from build123d import *

# Parameters (mm, degrees)
F0_R     = 2.1
F1_DEPTH = 19
F2_R     = 9.5
F3_DEPTH = 29.001
F4_R     = 5
F5_DEPTH = 38.001
F6_W     = 74.916892
F6_H     = 3.990418
F7_DEPTH = 29.001
F8_R     = 5
F9_DEPTH = 38.001


with BuildPart() as f1:
    # F0 (on Top) → F1 (new body)
    with BuildSketch(Plane.XY):
        Polygon((14, 14.5), (-14, 14.5), (-19, 9.5), (-19, -14.5), (19, -14.5), (19, 9.5), align=None)
        with Locations((-13, -9.8)):
            Circle(F0_R, mode=Mode.SUBTRACT)
        with Locations((13, -9.8)):
            Circle(F0_R, mode=Mode.SUBTRACT)
        with Locations((-13, 8.2)):
            Circle(F0_R, mode=Mode.SUBTRACT)
        with Locations((13, 8.2)):
            Circle(F0_R, mode=Mode.SUBTRACT)
    extrude(amount=F1_DEPTH)

    # F2 (on face) → F3 (cut, through all)
    with BuildSketch(Plane.XZ.offset(14.5)):
        with Locations((0, 16.5)):
            Circle(F2_R)
    extrude(amount=-F3_DEPTH, mode=Mode.SUBTRACT)

    # F4 (on face) → F5 (cut, through all)
    with BuildSketch(Plane.YZ.offset(19)):
        with Locations((-0.8, 0.2)):
            Circle(F4_R)
    extrude(amount=-F5_DEPTH, mode=Mode.SUBTRACT)

    # F6 (on face) → F7 (cut, through all)
    with BuildSketch(Plane.XZ.offset(14.5)):
        with Locations((0.39847, 18.995209)):
            Rectangle(F6_W, F6_H)
    extrude(amount=-F7_DEPTH, mode=Mode.SUBTRACT)

    # F8 (on face) → F9 (cut, through all)
    with BuildSketch(Plane(origin=(-19, 0, 0), x_dir=(0, -1, 0), z_dir=(-1, 0, 0))):
        with Locations((0.8, 0.7)):
            Circle(F8_R)
    extrude(amount=-F9_DEPTH, mode=Mode.SUBTRACT)


solid = f1.part
Part model, mm, in its own coordinate system. Round coordinates to 2 decimals unless told otherwise and drop trailing zeros. Write each loop counter-clockwise with the first axis right and the second up, starting at its lowest first coordinate (ties: lowest second). Pieces come first, ordered by that corner, then holes. Notation, with made-up numbers: M 33,-15 L 65,-15 A15 ccw 65,8 Z; hole C 30.5,-21.75 d6. An arc over 180 degrees is marked long. Return JSON: item names as keys, results as strings. Group by question number.
(1) Saw through at B-B on y = -9.8. Write the cut outline in (x, z), then the cut area to 3 significant figures.
(2) Saw through at A-A on x = 13. Write the cut outline in (y, z), then the cut area to 3 significant figures.
(3) Saw through at C-C on z = 14.25. Write the cut outline in (x, y).
(4) Two-plate mould, pull along Y, no slides. Class faces 1 (the face through (14, 0, 17)), 2 (the face through (0, 14.5, 6)), 3 (the face through (10.9, 8.29, 8.38)): +Y half, -Y half, draft (parallel to the pull), parting line (faces both ways), or undercut.
(5) Saw through at D-D on y = 12.25. Write the cut outline in (x, z).
(6) Pin check, flat tips, straight feed: pin 1 Ø10 at (x, y) = (3, -10) entering from +Z; pin 2 Ø8 at (x, y) = (8.5, -9) entering from +Z. Stop position of each tip, or through.
(7) Drill centre lines: probe 1 along Y at (x, z) = (-13, 10.25); probe 2 along X at (y, z) = (8, 1); probe 3 along X at (y, z) = (8.2, 12). Where is each one in solid material? Low to high.
Returned:
{
 "1": {"outline": "M -19,0 L -15.1,0 L -15.1,17 L -19,17 Z; M -10.9,0 L 10.9,0 L 10.9,17 L 9.49,17 A9.5 cw long -9.49,17 L -10.9,17 Z; M 15.1,0 L 19,0 L 19,17 L 15.1,17 Z", "area": "352 mm²"},
 "2": {"outline": "M -14.5,0 L -11.9,0 L -11.9,17 L -14.5,17 Z; M -7.7,0 L -5.8,0 A5 cw -5.79,0.45 A5 cw long 4.19,0.45 A5 cw 4.2,0 L 6.1,0 L 6.1,17 L -7.7,17 Z; M 10.3,0 L 14.5,0 L 14.5,17 L 10.3,17 Z", "area": "304 mm²"},
 "3": {"outline": "M -19,-14.5 L -9.23,-14.5 L -9.23,14.5 L -14,14.5 L -19,9.5 Z; M 9.23,-14.5 L 19,-14.5 L 19,9.5 L 14,14.5 L 9.23,14.5 Z; hole C -13,-9.8 d4.2; hole C -13,8.2 d4.2; hole C 13,-9.8 d4.2; hole C 13,8.2 d4.2"},
 "4": {"face 1": "draft", "face 2": "+Y half", "face 3": "undercut"},
 "5": {"outline": "M -16.25,0 L 16.25,0 L 16.25,17 L 9.49,17 A9.5 cw long -9.49,17 L -16.25,17 Z"},
 "6": {"pin 1": "z = 11.38", "pin 2": "z = 17"},
 "7": {"probe 1": "-14.5 to -11.9, -7.7 to 6.1, 10.3 to 14.5", "probe 2": "-19 to -15.09, -10.91 to 10.91, 15.09 to 19", "probe 3": "-19 to -15.1, -10.9 to -8.37, 8.37 to 10.9, 15.1 to 19"}
}
